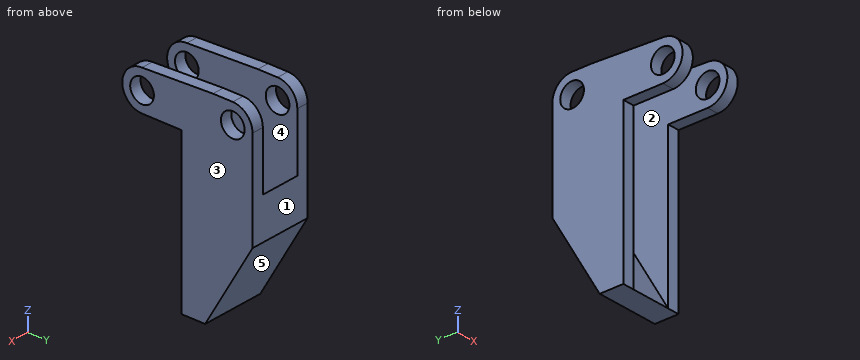
Autodesk Inventor part; units mm, degrees
ref_plane "工作平面2" through (0, 50, 27.1795) normal (0, 0.8660254, -0.5) x (1, 0, 0)
ref_plane "YZ Plane" through (0, 0, 0) normal (1, 0, 0) x (0, 1, 0)
ref_plane "XZ Plane" through (0, 0, 0) normal (0, 1, 0) x (-1, 0, 0)
sketch "草图1" plane through (0, 0, 0) normal (1, 0, 0) x (0, 1, 0)
  circle A0 centre (0, 0) radius 15
  arc A1 (0, 25) -> (0, -25) centre (0, 0) ccw
  line L0 (0, -25) -> (50, -25)
  line L1 (50, -25) -> (50, -225)
  line L2 (50, -225) -> (80, -225)
  line L3 (80, -225) -> (140, -121.077)
  line L4 (140, -121.077) -> (140, 28.923)
  line L5 (140, 28.923) -> (90, 28.923)
  line L6 (90, 28.923) -> (0, 25)
  dimension "d0" = 30
  dimension "d1" = 50
  dimension "d2" = 50
  dimension "d4" = 200
  dimension "d5" = 30
  dimension "d6" = 30
  dimension "d7" = 120
  dimension "d8" = 150
  dimension "d9" = 50
extrude "拉伸1" add sketch "草图1" along normal mid plane 80
sketch "草图2" plane through (-40, 50, -225) normal (0, -1, 0) x (1, 0, 0)
  line L0 (80, 0) -> (0, 0)
  line L1 (40, 0) -> (40, 253.923)
  line L2 (80, 253.923) -> (0, 253.923)
  line L3 (15, -693.1323) -> (65, -693.1323)
  line L4 (65, -693.1323) -> (65, 466.9493)
  line L5 (65, 466.9493) -> (15, 466.9493)
  line L6 (15, 466.9493) -> (15, -693.1323)
  line L7 (15, -693.1323) -> (65, 466.9493) construction
  line L8 (65, -693.1323) -> (15, 466.9493) construction
  point P0 (40, 225)
  point P1 (40, -113.0915)
  dimension "d12" = 50
extrude "拉伸2" cut sketch "草图2" along normal through all
ref_plane "工作平面2" through (0, 50, 27.1795) normal (0, 0.8660254, -0.5) x (1, 0, 0)
sketch "草图3" plane through (0, 50, 27.1795) normal (0, 0.8660254, -0.5) x (1, 0, 0)
  line L0 (25, -307.1385) -> (-25, -307.1385)
  line L1 (-25, -307.1385) -> (-25, 307.1385)
  line L2 (-25, 307.1385) -> (25, 307.1385)
  line L3 (25, 307.1385) -> (25, -307.1385)
  line L4 (-25, 0) -> (25, 0)
  line L5 (25, -307.1385) -> (-25, 307.1385) construction
  line L6 (-25, -307.1385) -> (25, 307.1385) construction
  point P0 (0, 48.5381)
  point P1 (0, 0)
  dimension "d16" = 50
extrude "拉伸3" cut sketch "草图3" along normal up to surface (126.0897 mm away)
fillet "圆角1" radius 25 2 edges at (-32.5, 140, 28.923) (32.5, 140, 28.923)
sketch "草图4" plane through (-40, 0, 0) normal (-1, 0, 0) x (0, 0, 1)
  line L0 (3.923, 140) -> (-121.077, 140)
  line L1 (28.923, 90) -> (28.923, 115)
  point P0 (0, 0)
  point P1 (3.923, 115)
  dimension "d27" = 25
  dimension "d28" = 25
hole "孔1" at (-40, 115, 3.923) direction (1, 0, 0) diameter 30 end through all
sketch "草图5" plane through (25, 0, -25) normal (-1, 0, 0) x (0, 0, 1)
  point P0 (25, 0)
properties part number "Finger" material "钢，高强度，低合金"
The listing builds one solid part. Answer for the finished solid, in the listing's coordinates (mm). Face numbers are marked on the shaded views. A direction names the side the tool comes from. Round coordinates to 2 decimals unless told otherwise and drop trailing zeros. Loops run counter-clockwise (first coordinate to the right, second up) from the corner with the lowest first, then second, coordinate; pieces in that order, holes last. Notation, with made-up numbers: M 23,53.25 L 53,53.25 A31 cw 53,77.25 Z; hole C -7.75,-2.5 d10. An arc over 180 degrees is marked long. Return JSON: item names as keys, results as strings.
Q1. Find section D-D, the plane z = -125.5. Determine the outline of the cut face in (x, y), plus the area to 3 significant figures.
Results list:
{"outline": "M -40,50 L -25,50 L -25,107.45 L 25,107.45 L 25,50 L 40,50 L 40,137.45 L -40,137.45 Z", "area": "4,120 mm2"}
Q2. Find section A-A, the plane z = -63. Determine the outline of the cut face in (x, y).
Results list:
{"outline": "M -40,50 L -25,50 L -25,140 L -40,140 Z; M 25,50 L 40,50 L 40,140 L 25,140 Z"}
Q3. Find section C-C, the plane y = 36.5. Determine the outline of the cut face in (x, z), plus the area to 3 significant figures.
Results list:
{"outline": "M -40,-25 L -25,-25 L -25,26.59 L -40,26.59 Z; M 25,-25 L 40,-25 L 40,26.59 L 25,26.59 Z", "area": "1,550 mm2"}
Q4. Find section B-B, the plane z = 0. Determine the outline of the cut face in (x, y).
Results list:
{"outline": "M -40,-25 L -25,-25 L -25,-15 L -40,-15 Z; M -40,15 L -25,15 L -25,100.52 L -40,100.52 Z; M -40,129.48 L -25,129.48 L -25,140 L -40,140 Z; M 25,-25 L 40,-25 L 40,-15 L 25,-15 Z; M 25,15 L 40,15 L 40,100.52 L 25,100.52 Z; M 25,129.48 L 40,129.48 L 40,140 L 25,140 Z"}
Q5. Each of these flat-tipped pins is pushed along its axis until it touches: pin 1 Ø8 at (x, z) = (-5, -117.5) entering from -Y; pin 2 Ø2 at (x, y) = (-5.5, 86) entering from -Z; pin 3 Ø4.5 at (x, z) = (-31, -85.5) entering from -Y. Where does it stop, or does it pass through?
Results list:
{"pin 1": "stops at y = 109.76", "pin 2": "stops at z = -216.34", "pin 3": "stops at y = 50"}
Q6. Find the intervals of material crossed by line 1 along Z through (x, y) = (35.5, 0); line 2 along X through (y, z) = (75, -88); line 3 along Y through (x, z) = (28.5, 0), in increasing order. Write a range as from..to.
Results list:
{"line 1": "z = -25..-15, 15..25", "line 2": "x = -40..-25, 25..40", "line 3": "y = -25..-15, 15..100.52, 129.48..140"}
Q7. The mould has two halves that part along X. Classify the marked faces 1, 2 and 3: released by +X, released by -X, zero draft, split by the parting line, or undercut.
Results list:
{"face 1": "zero draft", "face 2": "undercut", "face 3": "released by +X"}
Q8. Which of the six approach directions +Z, -Z, +X, -X, +Y, -Y give full straight-line access (tool end or side, diameter ignored) to the marked faces 4 and 5?
Results list:
{"face 4": "+Z, -Y", "face 5": "-Z, +X, -X, +Y"}
